Read the model definition and answer for the solid it produces. Units are mm, in the model's axes. A direction names the side the tool comes from. Coordinates: 2 decimals unless noted, no trailing zeros. Order: outer loops, then holes, each group sorted by start corner. A loop starts at its lowest first (then second) coordinate and runs counter-clockwise, first axis right, second up. Notation, with made-up numbers: (82.25, 48) -> (132.25, 48) arc R33 ccw to (132.25, 77) -> close; hole circle Ø9 at (-22, 86). An arc over 180 degrees is marked (long way). Use CSV: the item, a comma, the result in double quotes.
```python
from build123d import *

# Parameters (mm, degrees)
F0_W     = 110
F0_H     = 10
F0_R     = 2.5
F1_DEPTH = 25
F2_T     = -2.5
F3_R     = 2


# Not quite as in the source:
# - a feature names something its author has since deleted; it is built from what else it names


with BuildPart() as f1:
    # F0 (on Front) → F1 (new body)
    with BuildSketch(Plane.XZ):
        Rectangle(F0_W, F0_H)
        with Locations((-30, 0)):
            Circle(F0_R, mode=Mode.SUBTRACT)
        with Locations((30, 0)):
            Circle(F0_R, mode=Mode.SUBTRACT)
    extrude(amount=-F1_DEPTH)

    # F2
    f2_openings = [f1.faces().sort_by_distance(p)[0] for p in [
        (0, 12.5, -5),
        (0, 25, 0),
        (0, 12.5, 5),
        (-32.5, 12.5, 0),
        (27.5, 12.5, 0),
    ]]
    offset(amount=F2_T, openings=f2_openings)

    # F3
    f3_edges = [f1.edges().sort_by_distance(p)[0] for p in [
        (-55, 0, 0),
        (55, 0, 0),
    ]]
    fillet(f3_edges, radius=F3_R)


solid = f1.part
```
Item 1: Find section A-A, the plane y = 7.5. Give the vertices of the cut face in (x, z), then the cut area to 3 significant figures.
Return value:
outline,"(-55, -5) -> (-52.5, -5) -> (-52.5, 5) -> (-55, 5) -> close; (52.5, -5) -> (55, -5) -> (55, 5) -> (52.5, 5) -> close"
area,"50.0 mm^2"
Item 2: Find section B-B, the plane x = -30. Give the vertices of the cut face in (y, z), then the cut area to 3 significant figures.
Return value:
outline,"(0, -5) -> (2.5, -5) -> (2.5, -2.5) -> (0, -2.5) -> close; (0, 2.5) -> (2.5, 2.5) -> (2.5, 5) -> (0, 5) -> close"
area,"12.5 mm^2"
Item 3: Straight lines are drawn through the part: line 1 along X through (y, z) = (18.5, 0.25); line 2 along Z through (x, y) = (30, 1.8); line 3 along Y through (x, z) = (-10, 0). For each, find the intervals that lie inside material, in ascending order.
Return value:
line 1,"x = -55 to -52.5, 52.5 to 55"
line 2,"z = -5 to -2.5, 2.5 to 5"
line 3,"y = 0 to 2.5"
Item 4: Each of these flat-tipped pins is pushed along its axis until it touches: P1, Ø10, axis at x = 6, y = 8.5, coming from the +Z side; P2, Ø1.5, axis at x = -19, z = -2, coming from the -Y side; P3, Ø3, axis at x = -8, z = 1, coming from the +Y side. Where does it stop, or does it pass through?
Return value:
P1,"passes through"
P2,"stops at y = 0"
P3,"stops at y = 2.5"
Item 5: The mould has two halves that part along X. Classify faces 1 (the flat face through (-1, 2.5, 0)), 2 (the flat face through (0, 2, 5)), 3 (the cylindrical face through (-54.43, 0.6, 0.07)): +X half, -X half, draft (parallel to the pull), parting line (faces both ways), or undercut.
Return value:
face 1,"undercut"
face 2,"draft"
face 3,"-X half"
Item 6: Find section C-C, the plane z = 0. Give the vertices of the cut face in (x, y).
Return value:
outline,"(-55, 2) arc R2 ccw to (-53, 0) -> (-32.5, 0) -> (-32.5, 2.5) -> (-52.5, 2.5) -> (-52.5, 25) -> (-55, 25) -> close; (-27.5, 0) -> (27.5, 0) -> (27.5, 2.5) -> (-27.5, 2.5) -> close; (32.5, 0) -> (53, 0) arc R2 ccw to (55, 2) -> (55, 25) -> (52.5, 25) -> (52.5, 2.5) -> (32.5, 2.5) -> close"
Item 7: Find section D-D, the plane x = -11. Give the vertices of the cut face in (y, z), then the cut area to 3 significant figures.
Return value:
outline,"(0, -5) -> (2.5, -5) -> (2.5, 5) -> (0, 5) -> close"
area,"25.0 mm^2"
Item 8: A tool of negligible diameter and unlimited length cuts with its end or side. For faces 4 (the cylindrical face through (54.4, 0.57, 0.07)), 5 (the flat face through (52.5, 14, 0)), from which of +Z, -Z, +X, -X, +Y, -Y can it reach the whole face along a straight path? Write none if from no direction.
Return value:
face 4,"+Z, -Z, +X, -Y"
face 5,"+Z, -Z, +Y"
